Check sheet for the modelled part. Datum: model origin and axes. Units: mm. A direction names the side the tool comes from. Coordinates: 2 decimals unless noted, no trailing zeros. Order: outer loops, then holes, each group sorted by start corner. A loop starts at its lowest first (then second) coordinate and runs counter-clockwise, first axis right, second up. Notation, with made-up numbers: (36.25, 89.5) -> (72.25, 89.5) arc R20 ccw to (72.25, 96.5) -> close; hole circle Ø1 at (-10.5, -25). An arc over 180 degrees is marked (long way). Put each result on its own line as item: value. Start each with the question number.
Autodesk Inventor part; units mm, degrees
ref_plane "YZ Plane" through (0, 0, 0) normal (1, 0, 0) x (0, 1, 0)
ref_plane "XZ Plane" through (0, 0, 0) normal (0, 1, 0) x (-1, 0, 0)
ref_plane "XY Plane" through (0, 0, 0) normal (0, 0, 1) x (1, 0, 0)
sketch "Sketch2" plane through (0, 0, 0) normal (0, 1, 0) x (-1, 0, 0)
  line L0 (0, 0) -> (20, 0)
  line L1 (20, 0) -> (20, -35)
  line L2 (20, -35) -> (0, -35)
  line L3 (0, -35) -> (0, 0)
  dimension "d0" = 35
  dimension "d1" = 20
extrude "Extrusion1" add sketch "Sketch2" along normal blind 8
sketch "Sketch3" plane through (0, 0, -35) normal (0, 0, -1) x (-1, 0, 0)
  line L0 (0, 0) -> (20, 0)
  line L1 (1.9454, 0) -> (-8.0206, 6.9783)
  line L2 (-8.0206, 6.9783) -> (-2.2848, 15.1698) construction
  line L3 (-2.2848, 15.1698) -> (7.9547, 8)
  line L4 (0, 8) -> (20, 8)
  arc A0 (-2.2848, 15.1698) -> (-8.0206, 6.9783) centre (-5.1527, 11.074) ccw
  circle A1 centre (-5.1527, 11.074) radius 2.5
  line L5 (0, 0) -> (0, 8) construction
  line L6 (-5.1527, 11.074) -> (0, 8) construction
  line L7 (1.9454, 0) -> (7.9547, 8)
  line L8 (-2.2848, 15.1698) -> (6.7994, 6.4619)
  dimension "d4" = 5
  dimension "d5" = 10
  dimension "d6" = 6
  dimension "d21" = 35
extrude "Extrusion2" add sketch "Sketch3" against normal up to surface (35 mm away) contours L1 A0 L8 L7
sketch "Sketch4" plane through (0, 0, -35) normal (0, 0, -1) x (-1, 0, 0)
  line L0 (-8.0206, 6.9783) -> (0, 1.3622)
  line L1 (-4.533, 4.5362) -> (4.5811, -1.8456)
  line L2 (4.5811, -1.8456) -> (-4.9445, -1.8456)
  line L3 (-4.9445, -1.8456) -> (-4.533, 4.5362)
  point P0 (0, 0)
  point P1 (0, 1.3622)
extrude "Extrusion3" cut sketch "Sketch4" against normal up to next
sketch "Sketch5" plane through (0, 8, 0) normal (0, 1, 0) x (1, 0, 0)
  line L0 (-5.1948, 35) -> (-20, 35) construction
  line L1 (-12, 35) -> (-12, 25) construction
  line L2 (-12, 25) -> (-12, 10) construction
  line L3 (-20, 35) -> (-20, 0) construction
  point P0 (0, 0)
  point P1 (-7.9547, 35)
  dimension "d11" = 10
  dimension "d12" = 15
  dimension "d13" = 8
hole "Hole1" at (-12, 8, -25) at (-12, 8, -10) direction (0, -1, 0) diameter 6 end through all countersink diameter 10 countersink angle 90
fillet "Fillet1" radius 5 1 edges at (-5.1948, 8, -17.5)
sketch "Sketch6" plane through (0, 0, 0) normal (0, -1, 0) x (1, 0, 0)
  line L0 (8.0206, 0) -> (-1.9454, 0)
  line L1 (-1.9454, 0) -> (16.0794, 0)
  line L2 (16.0794, 0) -> (16.0794, -6.6)
  line L3 (16.0794, -6.6) -> (-1.9454, -6.6)
  line L4 (-1.9454, -6.6) -> (-1.9454, 0)
  point P0 (0, 0)
  dimension "d23" = 6.6
extrude "Extrusion4" cut sketch "Sketch6" against normal up to next
fillet "Fillet2" radius 5 1 edges at (-1.9454, 11.1148, -3.3)
pattern_linear "Rectangular Pattern1" count 3 spacing 11.6 along (0, 0, -1) of "Extrusion4", "Fillet2"
properties part number "halfhinge"
1) Sectioned sample at A-A (x = -12). Record the boundary of the cut face in (y, z), plus the area to 3 significant figures.
2) Sectioned sample at C-C (x = 6). Record the boundary of the cut face in (y, z).
3) Mould release check, pull along Y, two halves, no side actions. Record for faces 6 (the cylindrical face through (7.137, 9.553, -9.135)), 7 (the flat face through (2, 10, -29.8)), 8 (the cylindrical face through (9.184, 14.031, -32.436)): +Y half, -Y half, draft (parallel to the pull), parting line (faces both ways), or undercut.
4) Access from +Z, -Z, +X, -X, +Y, -Y to the whole of each face (thin tool, end or side, straight path). Record for faces 1 (the flat face through (4, 8, -6.6)), 2 (the flat face through (-1.945, 1, -3)), 3 (the flat face through (-15, 8, -17)), 4 (the flat face through (-1.945, 1, -27)), 5 (the flat face through (2, 10, -23.2)).
5) Gauge pin test, flat ends, axial feed: pin 1 (1.5 mm diameter, centred on y = 1, z = -28, fed in from +X); pin 2 (1 mm diameter, centred on x = 4, z = -10, fed in from +Y); pin 3 (6.5 mm diameter, centred on x = -15.5, z = -14, fed in from +Y). Record the tip position at first contact, or that the pin passes through.
6) Sectioned sample at D-D (z = -10). State how many separate pieces and enclosed holes the cut face has, plus the area to 3 significant figures.
7) Sectioned sample at B-B (y = 11.5). Record the boundary of the cut face in (x, z), plus the area to 3 significant figures.
8) Scan lines: line 1 along Z through (x, y) = (-12, 3.4); line 2 along Z through (x, y) = (1.5, 8.25); line 3 along Y through (x, z) = (-9, -31). Record each from-to range of solid material in increasing order. Write a range as [from, to].
Entries:
1. outline: (0, -35) -> (8, -35) -> (8, -30) -> (6, -28) -> (0, -28) -> close; (0, -22) -> (6, -22) -> (8, -20) -> (8, -15) -> (6, -13) -> (0, -13) -> close; (0, -7) -> (6, -7) -> (8, -5) -> (8, 0) -> (0, 0) -> close
1. area: 176 mm2
2. outline: (5.56, -35) -> (8.72, -35) -> (8.72, -29.8) -> (5.56, -29.8) -> close; (5.56, -23.2) -> (8.72, -23.2) -> (8.72, -18.2) -> (5.56, -18.2) -> close; (5.56, -11.6) -> (8.72, -11.6) -> (8.72, -6.6) -> (5.56, -6.6) -> close; (13.43, -35) -> (16, -35) -> (16, -29.8) -> (13.43, -29.8) -> close; (13.43, -23.2) -> (16, -23.2) -> (16, -18.2) -> (13.43, -18.2) -> close; (13.43, -11.6) -> (16, -11.6) -> (16, -6.6) -> (13.43, -6.6) -> close
3. face 6: undercut
3. face 7: draft
3. face 8: parting line
4. face 1: +Z, +X, +Y
4. face 2: +Z, +X, +Y, -Y
4. face 3: +Z, -Z, -X, +Y
4. face 4: +X, +Y, -Y
4. face 5: +X, +Y
5. pin 1: stops at x = -1.95
5. pin 2: stops at y = 16.03
5. pin 3: stops at y = 8
6. separate pieces: 2
6. enclosed holes: 1
6. area: 202 mm2
7. outline: (-1.54, -35) -> (2.69, -35) -> (2.69, -29.8) -> (-1.54, -29.8) -> close; (-1.54, -23.2) -> (2.69, -23.2) -> (2.69, -18.2) -> (-1.54, -18.2) -> close; (-1.54, -11.6) -> (2.69, -11.6) -> (2.69, -6.6) -> (-1.54, -6.6) -> close; (7.62, -35) -> (10.13, -35) -> (10.13, -29.8) -> (7.62, -29.8) -> close; (7.62, -23.2) -> (10.13, -23.2) -> (10.13, -18.2) -> (7.62, -18.2) -> close; (7.62, -11.6) -> (10.13, -11.6) -> (10.13, -6.6) -> (7.62, -6.6) -> close
7. area: 103 mm2
8. line 1: z = [-35, -28], [-22, -13], [-7, 0]
8. line 2: z = [-35, -29.8], [-23.2, -18.2], [-11.6, -6.6]
8. line 3: y = [0, 8]
